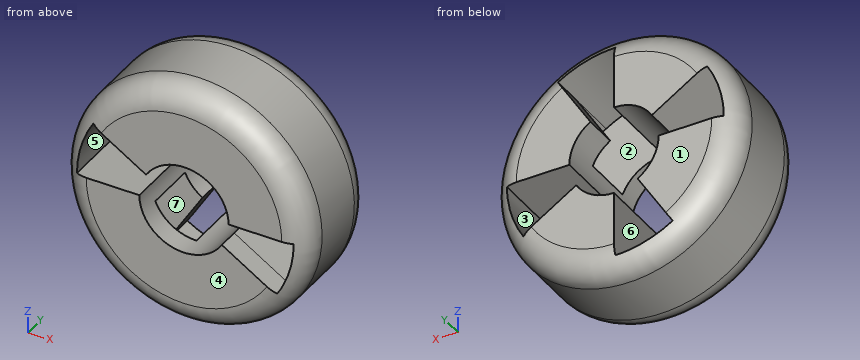
```python
from build123d import *

# Parameters (mm, degrees)
SKETCH2_W          = 9.25
SKETCH2_H          = 12.5
CUT_EXTRUDE1_DEPTH = 10
CIRPATTERN1_COUNT  = 4
CUT_EXTRUDE2_DEPTH = 10
CUT_EXTRUDE3_START = 6
CUT_EXTRUDE3_DEPTH = 6
CIRPATTERN2_COUNT  = 2
FILLET1_R          = 3


with BuildPart() as part:
    # Sketch2 → Revolve1 (revolve)
    with BuildSketch(Plane(origin=(0, 0, 0), x_dir=(0, 0, -1), z_dir=(1, 0, 0))):
        with Locations((-9.875, 6.25)):
            Rectangle(SKETCH2_W, SKETCH2_H)
    revolve(axis=Axis((0, 31, 0), (0, -1, 0)))

    # Sketch3 → Cut-Extrude1 (cut)
    with BuildSketch(Plane(origin=(0, 12.5, 0), x_dir=(1, 0, 0), z_dir=(0, 1, 0))):
        with BuildLine():
            Line((-6.756470619, 10.812613226), (0, 0))
            Line((0, 0), (0, 12.75))
            ThreePointArc((0, 12.75), (-3.514376287, 12.256086623), (-6.756470619, 10.812613226))
        make_face()
    cut_extrude1 = extrude(amount=-CUT_EXTRUDE1_DEPTH, mode=Mode.SUBTRACT)

    # CirPattern1: Cut-Extrude1 ×4 about axis
    cirpattern1_axis = Axis((0, 12.5, 0), (0, 1, 0))
    for i in range(1, CIRPATTERN1_COUNT):
        add(cut_extrude1.rotate(cirpattern1_axis, i * 360 / CIRPATTERN1_COUNT), mode=Mode.SUBTRACT)

    # Sketch4 → Cut-Extrude2 (cut)
    with BuildSketch(Plane(origin=(0, 2.5, 0), x_dir=(1, 0, 0), z_dir=(0, 1, 0))):
        with BuildLine():
            Line((5.25, 0), (12.75, 0))
            ThreePointArc((12.75, 0), (12.256086623, 3.514376287), (10.812613226, 6.756470619))
            Line((10.812613226, 6.756470619), (4.452252505, 2.782076137))
            ThreePointArc((4.452252505, 2.782076137), (5.046623904, 1.447096118), (5.25, 0))
        make_face()
        with BuildLine():
            Line((-5.25, 0), (-12.75, 0))
            ThreePointArc((-12.75, 0), (-12.256086623, -3.514376287), (-10.812613226, -6.756470619))
            Line((-10.812613226, -6.756470619), (-4.452252505, -2.782076137))
            ThreePointArc((-4.452252505, -2.782076137), (-5.046623904, -1.447096118), (-5.25, 0))
        make_face()
    extrude(amount=-CUT_EXTRUDE2_DEPTH, mode=Mode.SUBTRACT)

    # Sketch5 → Cut-Extrude3 (cut)
    with BuildSketch(Plane(origin=(0, 2.5, 0), x_dir=(1, 0, 0), z_dir=(0, 1, 0)).offset(CUT_EXTRUDE3_START)):
        with BuildLine():
            Line((0, 0), (-6.756470619, 10.812613226))
            ThreePointArc((-6.756470619, 10.812613226), (-9.695176061, 8.280462616), (-11.736436882, 4.981821888))
            Line((-11.736436882, 4.981821888), (0, 0))
        make_face()
    cut_extrude3 = extrude(amount=-CUT_EXTRUDE3_DEPTH, mode=Mode.SUBTRACT)

    # CirPattern2: Cut-Extrude3 ×2 about axis
    cirpattern2_axis = Axis((0, 12.5, 0), (0, 1, 0))
    for i in range(1, CIRPATTERN2_COUNT):
        add(cut_extrude3.rotate(cirpattern2_axis, i * 360 / CIRPATTERN2_COUNT), mode=Mode.SUBTRACT)

    # Fillet1
    # the kernel refuses this fillet: 3 mm, written as the material it takes off along each edge
    with BuildSketch(Plane(origin=(0, 12.5, 0), x_dir=(0, 0, 1), z_dir=(1, 0, 0))) as fillet1_piece_1:
        with BuildLine():
            CenterArc((14.5 - FILLET1_R, FILLET1_R), FILLET1_R, 270, 90)
            Line((14.5, FILLET1_R), (14.5, 0))
            Line((14.5, 0), (14.5 - FILLET1_R, 0))
        make_face()
    revolve(axis=Axis((0, 12.5, 0), (0, -1, 0)), mode=Mode.SUBTRACT)
    with BuildSketch(Plane(origin=(0, 0, 0), x_dir=(0, 0, 1), z_dir=(1, 0, 0))) as fillet1_piece_2:
        with BuildLine():
            CenterArc((14.5 - FILLET1_R, -FILLET1_R), FILLET1_R, 360, 90)
            Line((14.5, -FILLET1_R), (14.5, 0))
            Line((14.5, 0), (14.5 - FILLET1_R, 0))
        make_face()
    revolve(axis=Axis((0, 0, 0), (0, -1, 0)), mode=Mode.SUBTRACT)


solid = part.part
```
Here's how the part is built. I have some questions about the finished solid (model axes, mm). Face numbers are marked on the shaded views. A direction names the side the tool comes from. Give positions to 0.01 mm unless a question says otherwise; leave off trailing zeros. Loops run counter-clockwise (first coordinate to the right, second up) from the corner with the lowest first, then second, coordinate; pieces in that order, holes last. Notation, with made-up numbers: M -1.75,87 L 20.25,87 A16 ccw 20.25,112 Z; hole C 52,-28 d1. An arc over 180 degrees is marked long. Put each result on its own line as item: value. Start each with the question number.
(1) I need wall thicknesses on line 1 along Z through (x, y) = (-8, 3); line 2 along X through (y, z) = (5.5, 8.5); line 3 along Z through (x, y) = (-10.75, 6). Which ranges of each line are inside material? Lowest first, please. Write a range as [from, to].
(2) Will these pins go through, and if not, where does the flat tip stop? pin 1 Ø2 at (x, z) = (2.5, 0) entering from -Y; pin 2 Ø4 at (x, y) = (8, 5) entering from -Z; pin 3 Ø3 at (y, z) = (1.5, -8) entering from +X; pin 4 Ø2 at (x, y) = (7.5, 7.5) entering from -Z.
(3) I want a section at C-C on y = 11. Please give me the cut outline in (x, z).
(4) For the marked faces 5, 6 and 7, which set-ups out of +Z, -Z, +X, -X, +Y, -Y let a thin tool reach every point of the face, with its end or its side?
(5) I want a section at A-A on y = 3.75. Please give me the cut outline in (x, z), then the cut area to 3 significant figures.
(6) If we mould it in two halves opening along Y, with no side actions, what happens to the marked faces 1, 2, 3 and 4? For each: +Y half, -Y half, draft (parallel to the pull), parting line (faces both ways), or undercut.
(7) I want a section at B-B on x = 10.25. State how many separate pieces and enclosed holes the cut face has, then the cut area to 3 significant figures.
Answer block:
1. line 1: [-12.09, -9.93], [-3.4, 0], [5, 12.09]
1. line 2: [-11.75, 0], [9.5, 11.75]
1. line 3: [-9.73, -6.86], [-4.56, 0], [6.72, 9.73]
2. pin 1: through
2. pin 2: z = -13.2
2. pin 3: x = 12.75
2. pin 4: z = -12.96
3. outline: C 0,0 d28.2; hole M -12.75,0 L -5.25,0 A5.25 ccw -2.78,-4.45 L -6.76,-10.81 A12.75 ccw 0,-12.75 L 0,-5.25 A5.25 ccw 4.45,-2.78 L 10.81,-6.76 A12.75 ccw 12.75,0 L 5.25,0 A5.25 ccw 2.78,4.45 L 6.76,10.81 A12.75 ccw 0,12.75 L 0,5.25 A5.25 ccw -4.45,2.78 L -10.81,6.76 A12.75 ccw Z
4. face 5: +Y, -Y
4. face 6: +Y
4. face 7: none
5. outline: C 0,0 d29; hole M -12.75,0 L -5.25,0 A5.25 ccw -4.83,-2.05 L -11.74,-4.98 A12.75 ccw 0,-12.75 L 0,-5.25 A5.25 ccw 4.45,-2.78 L 10.81,-6.76 A12.75 ccw 12.75,0 L 5.25,0 A5.25 ccw 4.83,2.05 L 11.74,4.98 A12.75 ccw 0,12.75 L 0,5.25 A5.25 ccw -4.45,2.78 L -10.81,6.76 A12.75 ccw Z
5. area: 341 mm^2
6. face 1: +Y half
6. face 2: undercut
6. face 3: draft
6. face 4: -Y half
7. separate pieces: 2
7. enclosed holes: 1
7. area: 145 mm^2
